The listing builds one solid part. Answer for the finished solid, in the listing's coordinates (mm). A direction names the side the tool comes from. Give positions to 0.01 mm unless a question says otherwise; leave off trailing zeros. Write each loop counter-clockwise with the first axis right and the second up, starting at its lowest first coordinate (ties: lowest second). Pieces come first, ordered by that corner, then holes.
```python
from build123d import *

# Parameters (mm, degrees)
SKETCH_1_W          = 54
SKETCH_1_H          = 72
EXTRUDE_1_DEPTH     = 2
CUT_EXTRUDE_1_DEPTH = 2
SKETCH_4_R          = 1.525
CUT_EXTRUDE_2_DEPTH = 10
CUT_EXTRUDE_3_DEPTH = 2
SKETCH_6_R          = 9
SKETCH_6_R_2        = 7
EXTRUDE_2_DEPTH     = 2
FILLET_1_R          = 1.1
FILLET_2_R          = 2


with BuildPart() as part:
    # 草图1 → 凸台-拉伸1 (new body)
    with BuildSketch(Plane.XY):
        Rectangle(SKETCH_1_W, SKETCH_1_H)
    extrude(amount=EXTRUDE_1_DEPTH)

    # 草图2 → 切除-拉伸1 (cut)
    with BuildSketch(Plane.XY.offset(2)):
        Polygon((-27, 2), (27, 25.105342179), (27, 36), (-27, 36), align=None)
    extrude(amount=-CUT_EXTRUDE_1_DEPTH, mode=Mode.SUBTRACT)

    # 草图4 → 切除-拉伸2 (cut)
    with BuildSketch(Plane.XY.offset(2)):
        with Locations((-9, -33)):
            Circle(SKETCH_4_R)
        with Locations((11, -33)):
            Circle(SKETCH_4_R)
        with Locations((2, -4)):
            Circle(SKETCH_4_R)
        with Locations((22, -4)):
            Circle(SKETCH_4_R)
    extrude(amount=-CUT_EXTRUDE_2_DEPTH, mode=Mode.SUBTRACT)

    # 草图5 → 切除-拉伸3 (cut)
    with BuildSketch(Plane.XY.offset(2)):
        with BuildLine():
            add(Edge.make_bspline(
                [(-23.397341502, -27.80348221), (-21.673234043, -24.952193686), (-18.841423513, -18.327485381), (-10.833901378, -11.756527748), (-1.499041268, -10.102711826), (9.981460044, -9.932321008), (18.81490672, -7.97288353), (24.483468669, -6.167126568)],
                knots=[0, 0, 0, 0, 0.178737613, 0.383542115, 0.520640135, 0.67991784, 1, 1, 1, 1], degree=3))
            add(Edge.make_bspline(
                [(-23.397341502, -27.80348221), (-13.158468218, -26.821678375), (0.76741254, -27.683363702), (15.176508339, -20.910209598), (20.355493831, -13.972924669), (22.163544803, -8.919372749), (24.483468669, -6.167126568)],
                knots=[0, 0, 0, 0, 0.548813094, 0.719371647, 0.81105697, 1, 1, 1, 1], degree=3))
        make_face()
    extrude(amount=-CUT_EXTRUDE_3_DEPTH, mode=Mode.SUBTRACT)

    # 草图6 → 凸台-拉伸2 (add)
    with BuildSketch(Plane.XY.offset(2)):
        with Locations((0.558156392, -17.980778356)):
            Circle(SKETCH_6_R)
        with Locations((0.558156392, -17.980778356)):
            Circle(SKETCH_6_R_2, mode=Mode.SUBTRACT)
    extrude(amount=-EXTRUDE_2_DEPTH)

    # 圆角1
    fillet_1_edges = [part.edges().sort_by_distance(p)[0] for p in [
        (6.982938033, -24.283331876, 1),
        (-2.733607094, -26.357191261, 1),
        (-23.397341502, -27.80348221, 1),
        (24.483468669, -6.167126568, 1),
        (-4.823851044, -10.767318995, 1),
        (4.597302123, -9.938061044, 1),
    ]]
    fillet(fillet_1_edges, radius=FILLET_1_R)

    # 圆角2
    fillet_2_edges = [part.edges().sort_by_distance(p)[0] for p in [
        (-27, 2, 1),
        (27, 25.105342179, 1),
        (27, -36, 1),
        (-27, -36, 1),
    ]]
    fillet(fillet_2_edges, radius=FILLET_2_R)


solid = part.part
```
Item 1: A cutting plane is placed at B-B, the plane x = 11. Count the separate pieces of the cut face and the enclosed holes in it, plus the area to 3 significant figures.
Conclusion:
separate pieces: 3
enclosed holes: 0
area: 75.6 mm2
Item 2: Which of the six approach directions +Z, -Z, +X, -X, +Y, -Y give full straight-line access (tool end or side, diameter ignored) to faces 1 (the face through (-1.137, 13.066, 1.014)), 2 (the face through (9.415, -16.384, 1.014))?
Conclusion:
face 1: +Z, -Z, -X, +Y
face 2: +Z, -Z
Item 3: This flat-tipped pin is pushed along its axis until it touches: P1, Ø1.8, axis at x = -9, y = -33, coming from the -Z side. Where does it stop, or does it pass through?
Conclusion:
P1: passes through
Item 4: Consider probe 1 along Y at (x, z) = (22, 1.45) (3 decimals); probe 2 along Y at (x, z) = (21.5, 1.2) (3 decimals); probe 3 along X at (y, z) = (-16.5, 0.85). Determine where each line is inside the solid, lowest interval first.
Conclusion:
probe 1: y = -36 to -9.933, -7.061 to -5.525, -2.475 to 22.966
probe 2: y = -36 to -10.876, -7.065 to -5.441, -2.559 to 22.752
probe 3: x = -27 to -16.06, -8.32 to -6.28, 7.4 to 9.44, 18.38 to 27
Item 5: Determine the mould class of faces 3 (the face through (26.4, -35.43, 1.01)), 4 (the face through (-26.43, -35.4, 1.01)), 5 (the face through (3.79, -24.19, 1.01)) for opening direction X: pulls with the +X half, pulls with the -X half, needs draft (parallel to the pull), parting line crosses it, or undercut.
Conclusion:
face 3: pulls with the +X half
face 4: pulls with the -X half
face 5: undercut
Item 6: A cutting plane is placed at A-A, the plane y = -4. Give the vertices of the cut face in (x, z) (3 decimals), plus the area to 3 significant figures.
Conclusion:
outline: (-27, 0) - (0.475, 0) - (0.475, 2) - (-27, 2) - close; (3.525, 0) - (20.475, 0) - (20.475, 2) - (3.525, 2) - close; (23.525, 0) - (27, 0) - (27, 2) - (23.525, 2) - close
area: 95.8 mm2
Item 7: A cutting plane is placed at D-D, the plane y = 7. Give the vertices of the cut face in (x, z).
Conclusion:
outline: (-15.31, 0) - (27, 0) - (27, 2) - (-15.31, 2) - close
